Verification items for the finished model (mm, model axes). A direction names the side the tool comes from. Round coordinates to 2 decimals unless told otherwise and drop trailing zeros. Order: outer loops, then holes, each group sorted by start corner. A loop starts at its lowest first (then second) coordinate and runs counter-clockwise, first axis right, second up. Notation, with made-up numbers: (-2.5, -33.5) -> (38.5, -33.5) arc R34 cw to (38.5, 0.5) -> close; hole circle Ø5 at (5.5, 44). An arc over 180 degrees is marked (long way). Put each result on its own line as item: value.
from build123d import *

# Parameters (mm, degrees)
F0_W     = 25
F0_H     = 40
F1_DEPTH = 25
F2_W     = 25
F2_H     = 40
F2_R     = 7.4574120062
F3_DEPTH = 9.5
F5_R     = 0.9656854249


# Not quite as in the source:
# - the program builds the solid bodies; features that only make, move or delete a surface that nothing else refers to are left out


with BuildPart() as f1:
    # F0 (on Top) → F1 (new body)
    with BuildSketch(Plane.XY):
        with Locations((0.5926040933, 1.8275822699)):
            Rectangle(F0_W, F0_H)
    extrude(amount=F1_DEPTH)

    # F2 (on face) → F3 (join)
    with BuildSketch(Plane.XY.offset(25)):
        with Locations((0.5926040933, 1.8275822699)):
            Rectangle(F2_W, F2_H)
        with Locations((0.1519261859, -0.08621795)):
            Circle(F2_R, mode=Mode.SUBTRACT)
    extrude(amount=F3_DEPTH)

    # F5
    f5_edges = [f1.edges().sort_by_distance(p)[0] for p in [
        (-7.305486, -0.086218, 34.5),
    ]]
    fillet(f5_edges, radius=F5_R)


solid = f1.part
Item 1: Gauge pin test, flat ends, axial feed: pin 1 Ø4.5 at (x, y) = (-1.5, 0.5) entering from +Z; pin 2 Ø5 at (x, y) = (0.5, -9) entering from -Z. Record the tip position at first contact, or that the pin passes through.
Check sheet entries:
pin 1: stops at z = 25
pin 2: stops at z = 0
Item 2: Section check A-A on z = 27. Record the boundary of the cut face in (x, y).
Check sheet entries:
outline: (-11.91, -18.17) -> (13.09, -18.17) -> (13.09, 21.83) -> (-11.91, 21.83) -> close; hole circle Ø14.91 at (0.15, -0.09)
Item 3: Release check for a two-part mould opening along X. For faces 3 (the flat face through (-11.907, 2, 17)), 4 (the flat face through (0, 0, 25)), 5 (the flat face through (6, 7, 34.5)) record: +X half, -X half, draft (parallel to the pull), parting line (faces both ways), or undercut.
Check sheet entries:
face 3: -X half
face 4: undercut
face 5: draft
Item 4: Material ranges on L1, parallel to Z at x = -2.5, y = -5.5; L2, parallel to Z at x = -7.5, y = 2, recorded low to high. Write a range as [from, to].
Check sheet entries:
L1: z = [0, 25]
L2: z = [0, 34.37]
Item 5: Tool access check on faces 1 (the flat face through (13.093, 2, 17)), 2 (the cylindrical face through (-1.465, -7.366, 29.207)). Record the directions out of +Z, -Z, +X, -X, +Y, -Y that give a thin tool (end or side, any length) a straight path to the whole face; none if there is none.
Check sheet entries:
face 1: +Z, -Z, +X, +Y, -Y
face 2: +Z
